from build123d import *

# Parameters (mm, degrees)
SCHIZZO2_R               = 5
TAGLIO_ESTRUSIONE1_DEPTH = 16
SMUSSO1_SIZE             = 1


with BuildPart() as part:
    # Schizzo1 → Rivoluzione1 (revolve)
    with BuildSketch(Plane.XY):
        Polygon((0, 0), (0, 11), (1, 11), (1, 8.9), (4, 8.9), (4, 11), (15, 11), (15, 8.9), (18, 8.9), (18, 11), (19, 11), (19, 0), align=None)
    revolve(axis=Axis((19, 0, 0), (-1, 0, 0)))

    # Schizzo2 → Taglio-Estrusione1 (cut)
    with BuildSketch(Plane(origin=(19, 0, 0), x_dir=(0, 0, -1), z_dir=(1, 0, 0))):
        with Locations(Location((0, 0, 0), (0, 0, 90))):
            Circle(SCHIZZO2_R)
    extrude(amount=-TAGLIO_ESTRUSIONE1_DEPTH, mode=Mode.SUBTRACT)

    # Smusso1
    smusso1_edges = [part.edges().sort_by_distance(p)[0] for p in [
        (0, -11, 0),
        (19, -11, 0),
    ]]
    chamfer(smusso1_edges, length=SMUSSO1_SIZE - 0.0001)  # a hair under: the kernel refuses the full size


solid = part.part
Can you work these out from the model? Positions are in its coordinate system, mm. A direction names the side the tool comes from. Give positions to 0.01 mm unless a question says otherwise; leave off trailing zeros. Order: outer loops, then holes, each group sorted by start corner. A loop starts at its lowest first (then second) coordinate and runs counter-clockwise, first axis right, second up. Notation, with made-up numbers: M 50,89 L 69,89 A11 cw 69,110 Z; hole C -39,86.5 d5. An arc over 180 degrees is marked long. One line per question, with ' | ' between items.
Item 1: We'd pull the mould along Z, two halves only. Please class faces 4 (the face through (3, 0, 0)), 5 (the face through (2.52, -1.93, 8.69)), 6 (the face through (18, 1, 9)): released by +Z, released by -Z, zero draft, split by the parting line, or undercut.
Answer block:
face 4: undercut | face 5: split by the parting line | face 6: zero draft
Item 2: I'm going to push flat-ended pins straight in: pin 1 Ø1.5 at (x, z) = (5, -8) entering from +Y; pin 2 Ø8 at (y, z) = (0, 0) entering from +X; pin 3 Ø3 at (x, y) = (3, 4.5) entering from +Z. Where does each tip first touch, or does it pass through?
Answer block:
pin 1: stops at y = 8.27 | pin 2: stops at x = 3 | pin 3: stops at z = 10.47
Item 3: Please list where these lines run through material, in increasing order: L1, parallel to X at y = -9.5, z = -0.5; L2, parallel to Z at x = 8.5, y = 0; L3, parallel to Z at x = 15.25, y = 0.
Answer block:
L1: x = 0 to 1, 4 to 15, 18 to 19 | L2: z = -11 to -5, 5 to 11 | L3: z = -8.9 to -5, 5 to 8.9
Item 4: Suppose I cut it at D-D, the plane x = 1.75. Write out the boundary of the cut face in (y, z), then the cut area to 3 significant figures.
Answer block:
outline: C 0,0 d17.8 | area: 249 mm2
Item 5: Suppose I cut it at C-C, the plane y = 9.5. Give the number of separate pieces and of enclosed holes in the cut face, then the cut area to 3 significant figures.
Answer block:
separate pieces: 3 | enclosed holes: 0 | area: 140 mm2
Item 6: For faces 1 (the face through (19, 2, -5)), 2 (the face through (1, -1, 9)), 3 (the face through (11.11, -1.08, -4.88)), which set-ups out of +Z, -Z, +X, -X, +Y, -Y let a thin tool reach every point of the face, with its end or its side?
Answer block:
face 1: +Z, -Z, +X, +Y, -Y | face 2: none | face 3: +X
